```python
from build123d import *

# Parameters (mm, degrees)
F0_W     = 101.6
F0_H     = 38.1
F1_DEPTH = 6.35
F3_DEPTH = 25.4
F4_R     = 19.05
F5_DEPTH = 69.85
F6_R     = 12.7
F7_DEPTH = 63.5
F8_R     = 4.7625
F9_DEPTH = 76.201


with BuildPart() as f1:
    # F0 (on Top) → F1 (new body)
    with BuildSketch(Plane.XY):
        with Locations((50.8, 19.05)):
            Rectangle(F0_W, F0_H)
    extrude(amount=F1_DEPTH)

    # F2 (on Top) → F3 (cut)
    with BuildSketch(Plane.XY):
        with BuildLine():
            Line((15.748, 28.702), (0, 28.702))
            Line((0, 28.702), (0, 9.398))
            Line((0, 9.398), (15.748, 9.398))
            ThreePointArc((15.748, 9.398), (25.4, 19.05), (15.748, 28.702))
        make_face()
        with BuildLine():
            Line((101.6, 9.398), (101.6, 28.702))
            Line((101.6, 28.702), (85.852, 28.702))
            ThreePointArc((85.852, 28.702), (76.2, 19.05), (85.852, 9.398))
            Line((85.852, 9.398), (101.6, 9.398))
        make_face()
    extrude(amount=F3_DEPTH, mode=Mode.SUBTRACT)

    # F4 (on face) → F5 (join)
    with BuildSketch(Plane.XY):
        with Locations((50.8, 19.05)):
            Circle(F4_R)
    extrude(amount=-F5_DEPTH)

    # F6 (on face) → F7 (cut)
    with BuildSketch(Plane.XY.offset(6.35)):
        with Locations((50.8, 19.05)):
            Circle(F6_R)
    extrude(amount=-F7_DEPTH, mode=Mode.SUBTRACT)

    # F8 (on face) → F9 (cut, through all)
    with BuildSketch(Plane(origin=(0, 0, -69.85), x_dir=(1, 0, 0), z_dir=(0, 0, -1))):
        with Locations((50.8, -19.05)):
            Circle(F8_R)
    extrude(amount=-F9_DEPTH, mode=Mode.SUBTRACT)


solid = f1.part
```
For this review, take the finished solid that the model builds, in its own axes (mm). A direction names the side the tool comes from. Round coordinates to 2 decimals unless told otherwise and drop trailing zeros. Write each loop counter-clockwise with the first axis right and the second up, starting at its lowest first coordinate (ties: lowest second). Pieces come first, ordered by that corner, then holes. Notation, with made-up numbers: (53, 42.5) - (84, 42.5) arc R38 cw to (84, 81.5) - close; hole circle Ø8 at (64.5, -36). An arc over 180 degrees is marked (long way). Use CSV: the item, a comma, the result in double quotes.
1) Wall thickness on line 1 along Y through (x, z) = (51, -27); line 2 along X through (y, z) = (19.05, -66.5); line 3 along X through (y, z) = (19.5, -9): over which ranges is each line inside the solid? List them lowest first. Write a range as from..to.
Conclusion:
line 1,"y = 0..6.35, 31.75..38.1"
line 2,"x = 31.75..46.04, 55.56..69.85"
line 3,"x = 31.76..38.11, 63.49..69.84"
2) Add section B-B on x = 17. Write out the cut boundary in (y, z).
Conclusion:
outline,"(0, 0) - (9.48, 0) - (9.48, 6.35) - (0, 6.35) - close; (28.62, 0) - (38.1, 0) - (38.1, 6.35) - (28.62, 6.35) - close"
3) Add section C-C on z = -42.5. Write out the cut boundary in (x, y).
Conclusion:
outline,"circle Ø38.1 at (50.8, 19.05); hole circle Ø25.4 at (50.8, 19.05)"
4) Clearance check with flat-ended pins moving along their axes: pin 1 Ø2 at (y, z) = (8.5, -20.5) entering from -X; pin 2 Ø3 at (x, y) = (22.5, 25.5) entering from -Z; pin 3 Ø12 at (y, z) = (9.5, -27.5) entering from +X. State where each tip first meets the part, or that it passes through.
Conclusion:
pin 1,"stops at x = 34.32"
pin 2,"stops at z = 0"
pin 3,"stops at x = 69.52"
5) The part is to be moulded in two halves that separate along Y. For faces 1 (the cylindrical face through (40.722, 11.322, -24.956)), 2 (the cylindrical face through (36.759, 31.925, -34.436)), 3 (the flat face through (55, 15, -69.85)), say which applies: pulls with the +Y half, pulls with the -Y half, needs draft (parallel to the pull), parting line crosses it, or undercut.
Conclusion:
face 1,"undercut"
face 2,"parting line crosses it"
face 3,"needs draft"
6) Add section A-A on y = 19.05. Write out the cut boundary in (x, z).
Conclusion:
outline,"(25.4, 0) - (31.75, 0) - (31.75, -69.85) - (46.04, -69.85) - (46.04, -57.15) - (38.1, -57.15) - (38.1, 6.35) - (25.4, 6.35) - close; (55.56, -69.85) - (69.85, -69.85) - (69.85, 0) - (76.2, 0) - (76.2, 6.35) - (63.5, 6.35) - (63.5, -57.15) - (55.56, -57.15) - close"
7) Add section D-D on x = 59. Write out the cut boundary in (y, z).
Conclusion:
outline,"(0, 0) - (1.86, 0) - (1.86, -69.85) - (36.24, -69.85) - (36.24, 0) - (38.1, 0) - (38.1, 6.35) - (28.75, 6.35) - (28.75, -57.15) - (9.35, -57.15) - (9.35, 6.35) - (0, 6.35) - close"
8) For faces 4 (the flat face through (8, 28.702, 3)), 5 (the flat face through (94, 9.398, 3)), 6 (the flat face through (56, 19, -57.15)), 7 (the flat face through (0, 5, 3)), list the 3-axis set-ups (+Z, -Z, +X, -X, +Y, -Y) from which the entire face can be reached by the end or side of a thin tool; tool diameter is ignored.
Conclusion:
face 4,"+Z, -Z, -X"
face 5,"+Z, -Z, +X"
face 6,"+Z"
face 7,"+Z, -Z, -X, +Y, -Y"
